Read the model definition and answer for the solid it produces. Units are mm, in the model's axes. Face numbers are marked on the shaded views. A direction names the side the tool comes from. Coordinates: 2 decimals unless noted, no trailing zeros. Loops run counter-clockwise (first coordinate to the right, second up) from the corner with the lowest first, then second, coordinate; pieces in that order, holes last. Notation, with made-up numbers: M 61,68.5 L 105,68.5 A15 ccw 105,79.5 Z; hole C 34.25,-0.5 d10. An arc over 180 degrees is marked long. One line per item, written item: value. Start each with the question number.
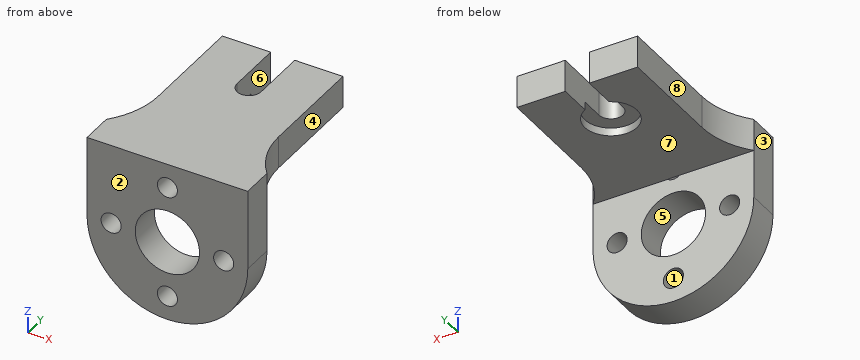
```python
from build123d import *

# Parameters (mm, degrees)
BOSS_EXTRUDE1_DEPTH = 4
SKETCH3_R           = 4
SKETCH3_R_2         = 1.25
CUT_EXTRUDE1_DEPTH  = 4
SKETCH4_W           = 20
SKETCH4_H           = 4
BOSS_EXTRUDE2_DEPTH = 20
SKETCH5_R           = 1.5
CUT_EXTRUDE2_DEPTH  = 30
SKETCH6_R           = 3.25
CUT_EXTRUDE3_DEPTH  = 1
SKETCH7_W           = 2.5
SKETCH7_H           = 20
CUT_EXTRUDE4_DEPTH  = 4
FILLET1_R           = 10


with BuildPart() as part:
    # Sketch1 → Boss-Extrude1 (new body)
    with BuildSketch(Plane(origin=(0, 0, 0), x_dir=(1, 0, 0), z_dir=(0, 1, 0))):
        with BuildLine():
            Line((-10, -10), (10, -10))
            Line((10, -10), (10, 0))
            ThreePointArc((10, 0), (0, 10), (-10, 0))
            Line((-10, 0), (-10, -10))
        make_face()
    extrude(amount=BOSS_EXTRUDE1_DEPTH)

    # Sketch3 → Cut-Extrude1 (cut)
    with BuildSketch(Plane(origin=(0, 4, 0), x_dir=(1, 0, 0), z_dir=(0, 1, 0))):
        with Locations(Location((0, 0, 0), (0, 0, 270))):
            Circle(SKETCH3_R)
        with Locations(Location((0, 7, 0), (0, 0, 270))):
            Circle(SKETCH3_R_2)
        with Locations(Location((7, 0, 0), (0, 0, 270))):
            Circle(SKETCH3_R_2)
        with Locations(Location((0, -7, 0), (0, 0, 270))):
            Circle(SKETCH3_R_2)
        with Locations(Location((-7, 0, 0), (0, 0, 270))):
            Circle(SKETCH3_R_2)
    extrude(amount=-CUT_EXTRUDE1_DEPTH, mode=Mode.SUBTRACT)

    # Sketch4 → Boss-Extrude2 (add)
    with BuildSketch(Plane(origin=(0, 4, 0), x_dir=(1, 0, 0), z_dir=(0, 1, 0))):
        with Locations((0, -8)):
            Rectangle(SKETCH4_W, SKETCH4_H)
    extrude(amount=BOSS_EXTRUDE2_DEPTH)

    # Sketch5 → Cut-Extrude2 (cut)
    with BuildSketch(Plane(origin=(0, 0, 6), x_dir=(-1, 0, 0), z_dir=(0, 0, -1))):
        with BuildLine():
            Line((-1.5, 24), (-1.5, 17))
            ThreePointArc((-1.5, 17), (0, 18.5), (1.5, 17))
            Line((1.5, 17), (1.5, 24))
            Line((1.5, 24), (-1.5, 24))
        make_face()
        with Locations((0, 17)):
            Circle(SKETCH5_R)
    extrude(amount=-CUT_EXTRUDE2_DEPTH, mode=Mode.SUBTRACT)

    # Sketch6 → Cut-Extrude3 (cut)
    with BuildSketch(Plane(origin=(0, 0, 6), x_dir=(-1, 0, 0), z_dir=(0, 0, -1))):
        with Locations((0, 17)):
            Circle(SKETCH6_R)
    extrude(amount=-CUT_EXTRUDE3_DEPTH, mode=Mode.SUBTRACT)

    # Sketch7 → Cut-Extrude4 (cut)
    with BuildSketch(Plane(origin=(0, 0, 6), x_dir=(-1, 0, 0), z_dir=(0, 0, -1))):
        with Locations((8.75, 14)):
            Rectangle(SKETCH7_W, SKETCH7_H)
        with Locations((-8.75, 14)):
            Rectangle(SKETCH7_W, SKETCH7_H)
    extrude(amount=-CUT_EXTRUDE4_DEPTH, mode=Mode.SUBTRACT)

    # Fillet1
    # the kernel refuses this fillet: 10 mm, written as the material it adds along each edge
    with BuildSketch(Plane(origin=(7.5, 4, 6), x_dir=(0, 1, 0), z_dir=(0, 0, 1))) as fillet1_piece_1:
        with BuildLine():
            CenterArc((6.614378278, -10), FILLET1_R, 90, 41.409622109)
            Line((0, -2.5), (0, 0))
            Line((0, 0), (6.614378278, 0))
        make_face()
    extrude(amount=4)
    with BuildSketch(Plane(origin=(-7.5, 4, 6), x_dir=(0, 1, 0), z_dir=(0, 0, 1))) as fillet1_piece_2:
        with BuildLine():
            CenterArc((6.614378278, 10), FILLET1_R, 228.590377891, 41.409622109)
            Line((0, 2.5), (0, 0))
            Line((0, 0), (6.614378278, 0))
        make_face()
    extrude(amount=4)


solid = part.part
```
1) Section A-A (x = 0) is taken. Determine the outline of the cut face in (y, z), then the cut area to 4 significant figures.
2) A tool of negligible diameter and unlimited length cuts with its end or side. For the marked faces 4, 5, 6, 7 and 8, from which of +Z, -Z, +X, -X, +Y, -Y can it reach the whole face along a straight path? Write none if from no direction.
3) Consider line 1 along X through (y, z) = (1.2, 0); line 2 along X through (y, z) = (10.25, 6.5); line 3 along Z through (x, y) = (-6.25, 7). Determine where each line is inside the solid, lowest interval first.
4) Section B-B (z = -2) is taken. Determine the outline of the cut face in (x, y), then the cut area to 3 significant figures.
5) Section D-D (z = 6.5) is taken. Determine the outline of the cut face in (x, y), then the cut area to 3 significant figures.
6) Section C-C (x = -7) is taken. Determine the outline of the cut face in (y, z).
7) Flat-ended cylindrical pins translate along their axes: pin 1 (3 mm diameter, centred on x = 5.5, y = 10.5, fed in from -Z); pin 2 (0.7 mm diameter, centred on x = -0.5, z = 7.5, fed in from -Y); pin 3 (4.5 mm diameter, centred on y = 21, z = 9, fed in from +X); pin 4 (1.5 mm diameter, centred on x = 0, z = -7, fed in from +Y). Find the tip coordinate at first contact, or state that the pin passes through.
8) For a pull along X with two mould halves and no side action, classify the marked faces 1, 2 and 3 as released by +X, released by -X, zero draft, split by the parting line, or undercut.
Results found:
1. outline: M 0,-10 L 4,-10 L 4,-8.25 L 0,-8.25 Z; M 0,-5.75 L 4,-5.75 L 4,-4 L 0,-4 Z; M 0,4 L 4,4 L 4,5.75 L 0,5.75 Z; M 0,8.25 L 4,8.25 L 4,6 L 13.75,6 L 13.75,7 L 15.5,7 L 15.5,10 L 0,10 Z
1. area: 72.25 mm²
2. face 4: +Z, -Z, +X, +Y
2. face 5: +Y, -Y
2. face 6: +Z, -Z, +Y
2. face 7: -Z, +X, -X, +Y
2. face 8: +Z, -Z, -X, +Y
3. line 1: x = -10 to -8.25, -5.75 to -4, 4 to 5.75, 8.25 to 10
3. line 2: x = -7.51 to 7.51
3. line 3: z = 6 to 10
4. outline: M -9.8,0 L -3.46,0 L -3.46,4 L -9.8,4 Z; M 3.46,0 L 9.8,0 L 9.8,4 L 3.46,4 Z
4. area: 50.7 mm²
5. outline: M -10,0 L -1.15,0 L -1.15,4 L 1.15,4 L 1.15,0 L 10,0 L 10,4 A10 cw 7.5,10.61 L 7.5,24 L 1.5,24 L 1.5,19.88 A3.25 cw long -1.5,19.88 L -1.5,24 L -7.5,24 L -7.5,10.61 A10 cw -10,4 Z
5. area: 336 mm²
6. outline: M 0,-7.14 L 4,-7.14 L 4,-1.25 L 0,-1.25 Z; M 0,1.25 L 4,1.25 L 4,6 L 24,6 L 24,10 L 0,10 Z
7. pin 1: stops at z = 6
7. pin 2: stops at y = 4
7. pin 3: stops at x = 7.5
7. pin 4: passes through
8. face 1: undercut
8. face 2: zero draft
8. face 3: released by -X
